Answer from the drawing. Dimensions are ordinates in mm from the lowest x, y and z of the part. Coordinates: 2 decimals unless noted, no trailing zeros. Write each loop counter-clockwise with the first axis right and the second up, starting at its lowest first coordinate (ties: lowest second). Pieces come first, ordered by that corner, then holes.
1) The part is cut by section B-B (x = 10). Determine the outline of the cut face in (y, z).
2) Find the intervals of material crossed by line 1 (X direction, y = 1.1, z = 10); line 2 (Z direction, x = 150, y = 0.4); line 3 (X direction, y = 0.45, z = 7.75), in increasing order.
3) The part is cut by section A-A (z = 10). Determine the outline of the cut face in (x, y), then the cut area to 3 significant figures.
4) This flat-tipped pin is pushed along its axis until it touches: pin 1 Ø3 at (x, z) = (150, 10) entering from +Y. Where does it stop, or does it pass through?
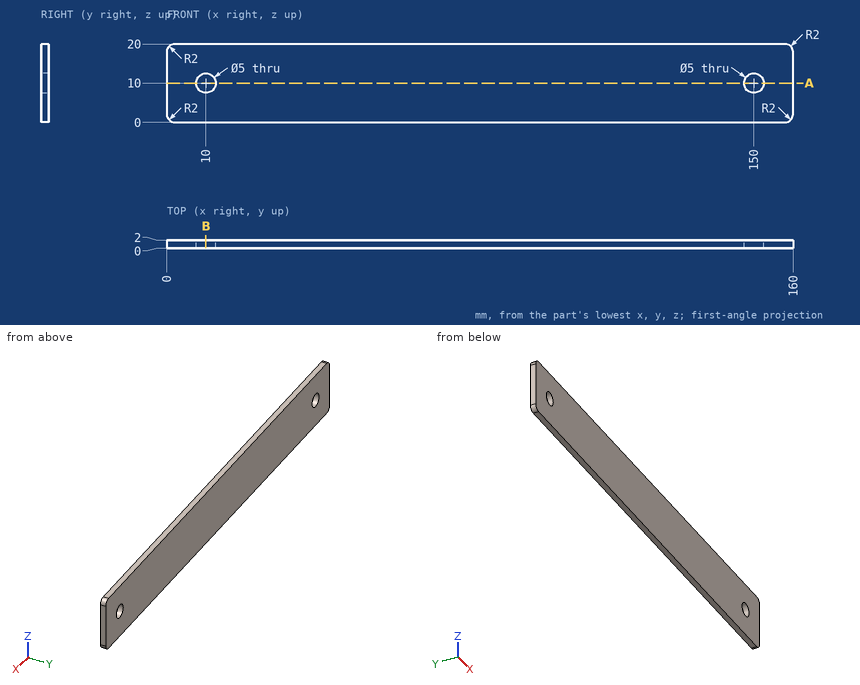
Reported:
1. outline: (0, 0) - (2, 0) - (2, 7.5) - (0, 7.5) - close; (0, 12.5) - (2, 12.5) - (2, 20) - (0, 20) - close
2. line 1: x = 0 to 7.5, 12.5 to 147.5, 152.5 to 160
2. line 2: z = 0 to 7.5, 12.5 to 20
2. line 3: x = 0 to 8.91, 11.09 to 148.91, 151.09 to 160
3. outline: (0, 0) - (7.5, 0) - (7.5, 2) - (0, 2) - close; (12.5, 0) - (147.5, 0) - (147.5, 2) - (12.5, 2) - close; (152.5, 0) - (160, 0) - (160, 2) - (152.5, 2) - close
3. area: 300 mm2
4. pin 1: passes through
